Build history of the part. All positions in model axes, mm. Face numbers are marked on the shaded views. A direction names the side the tool comes from. Give positions to 0.01 mm unless a question says otherwise; leave off trailing zeros. Order: outer loops, then holes, each group sorted by start corner. A loop starts at its lowest first (then second) coordinate and runs counter-clockwise, first axis right, second up. Notation, with made-up numbers: (19.5, -35) - (34.5, -35) arc R9 cw to (34.5, -21) - close; hole circle Ø9 at (30.25, 30.25). An arc over 180 degrees is marked (long way). Use a Markdown table: item, result.
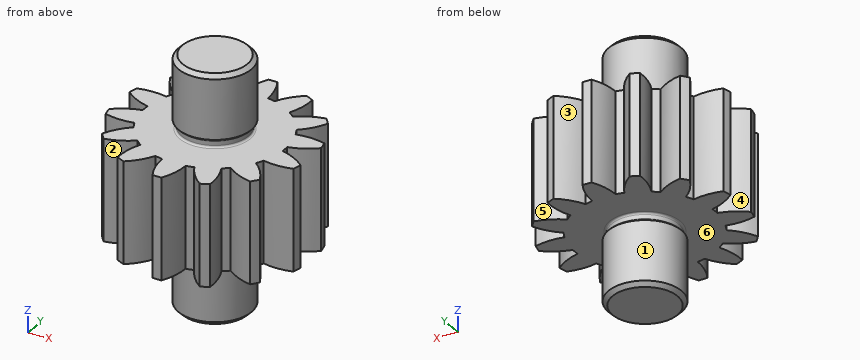
Autodesk Inventor part; units mm, degrees
ref_plane "工作平面1" through (0, -3, 0) normal (0, 1, 0) x (-1, 0, 0)
ref_plane "YZ Plane" through (0, 0, 0) normal (1, 0, 0) x (0, 1, 0)
ref_plane "XY Plane" through (0, 0, 0) normal (0, 0, 1) x (1, 0, 0)
sketch "草图1" plane through (0, 0, 0) normal (0, 0, 1) x (1, 0, 0)
  circle A0 centre (0, 0) radius 9
  dimension "d0" = 18
extrude "拉伸1" add sketch "草图1" along normal blind 16
sketch "草图2" plane through (0, 0, 16) normal (0, 0, 1) x (1, 0, 0)
  circle A0 centre (0, 0) radius 9
  circle A1 centre (0, 0) radius 8.2
  dimension "d3" = 16.4
extrude "拉伸2" add sketch "草图2" along normal blind 2 contours A1
sketch "草图3" plane through (0, 0, 18) normal (0, 0, 1) x (1, 0, 0)
  circle A0 centre (0, 0) radius 8.2
  circle A1 centre (0, 0) radius 17.25
  dimension "d6" = 34.5
extrude "拉伸3" add sketch "草图3" along normal blind 25 contours A0 | A1
sketch "草图4" plane through (0, 0, 43) normal (0, 0, 1) x (1, 0, 0)
  circle A0 centre (0, 0) radius 8.2
  circle A1 centre (0, 0) radius 8.2
extrude "拉伸4" add sketch "草图4" along normal blind 2
sketch "草图5" plane through (0, 0, 45) normal (0, 0, 1) x (1, 0, 0)
  circle A0 centre (0, 0) radius 8.2
  circle A1 centre (0, 0) radius 9
  dimension "d11" = 18
extrude "拉伸5" add sketch "草图5" along normal blind 16 contours A0 | A1
fillet "圆角2" radius 0.5 2 edges at (-8.2, 0, 16) (-8.2, 0, 18)
chamfer "倒角2" distance 0.3 angle 45 1 edges at (-9, 0, 16)
chamfer "倒角3" distance 0.3 angle 45 1 edges at (-9, 0, 45)
fillet "圆角4" radius 0.5 2 edges at (-8.2, 0, 45) (-8.2, 0, 43)
chamfer "倒角5" distance 1 angle 45 1 edges at (-9, 0, 0)
ref_plane "工作平面1" through (0, -3, 0) normal (0, 1, 0) x (-1, 0, 0)
sketch "草图13" plane through (0, 0, 18) normal (0, 0, -1) x (-1, 0, 0)
  circle A0 centre (0, 0) radius 17.25
  circle A1 centre (0, 0) radius 8.7
  circle A2 centre (0, 0) radius 21
  circle A3 centre (0, 0) radius 24
  circle A4 centre (0, 0) radius 17.25
  arc A5 (-1.1074, 23.9744) -> (-2.8831, 17.0074) centre (11.9993, 16.9242) ccw
  line L0 (0, 0) -> (0, 27.2026) construction
  arc A6 (2.8831, 17.0074) -> (1.1074, 23.9744) centre (-11.9993, 16.9242) ccw
  arc A7 (1.1074, 23.9744) -> (-1.1074, 23.9744) centre (0, 0) ccw
  point P0 (-2.3513, 20.868)
  point P1 (2.3513, 20.868)
  point P2 (2.8831, 17.0074)
  point P3 (-2.8831, 17.0074)
  dimension "d68" = 42
  dimension "d69" = 48
  dimension "d70" = 12.857
extrude "拉伸11" add sketch "草图13" against normal up to surface (25 mm away) contours A0 A5 A2 A6 | A2 A5 A3 A6 picked at (-0.2617, 18.4771) picked at (0.1231, 21.9893)
pattern_circular "环形阵列1" count 14 over 360 about axis through (0, 0, 18) along (0, 0, 1) of "拉伸11"
chamfer "倒角6" distance 1 angle 45 1 edges at (-9, 0, 61)
properties part number "主动齿轮轴" material "钢"
1) Tool access for the marked faces 1, 2 and 3: list every direction of +Z, -Z, +X, -X, +Y, -Y with a clear straight run to the whole face (end or side of a thin tool).
Computed:
| item | result |
|---|---|
| face 1 | -Z |
| face 2 | +Z, -Z, -Y |
| face 3 | +Z, -Z, +Y |
2) Slice it at B-B (x = 14). Write the cut outline in (y, z).
Computed:
| item | result |
|---|---|
| outline | (-14.45, 18) - (14.45, 18) - (14.45, 43) - (-14.45, 43) - close |
3) Pin check, flat tips, straight feed: P1, Ø1, axis at y = 1.5, z = 10, coming from the +X side; P2, Ø14, axis at x = 8.5, y = 2, coming from the +Z side; P3, Ø1.5, axis at x = -8.5, y = 17.5, coming from the -Z side; P4, Ø10, axis at x = 5.5, z = 51.5, coming from the -Y side. Stop position of each tip, or through.
Computed:
| item | result |
|---|---|
| P1 | stops at x = 8.94 |
| P2 | stops at z = 61 |
| P3 | stops at z = 18 |
| P4 | stops at y = -8.99 |
4) Two-plate mould, pull along X, no slides. Class the marked faces 4, 5 and 6: +X half, -X half, draft (parallel to the pull), parting line (faces both ways), or undercut.
Computed:
| item | result |
|---|---|
| face 4 | -X half |
| face 5 | undercut |
| face 6 | draft |
5) Wall check: line 1 (Y direction, x = -19, z = 38); line 2 (X direction, y = 18, z = 19); line 3 (Z direction, x = -18.5, y = 14.5). Give the ranges that are in metal, low to high. Write a range as from..to.
Computed:
| item | result |
|---|---|
| line 1 | y = -14.66..-13.16, -6.95..-1.51, 1.51..6.95, 13.16..14.66 |
| line 2 | x = -11.21..-5.58, -2.84..2.84, 5.58..11.21 |
| line 3 | z = 18..43 |
6) Slice it at A-A (z = 56.5). Write the cut outline in (x, y).
Computed:
| item | result |
|---|---|
| outline | circle Ø18 at (0, 0) |
